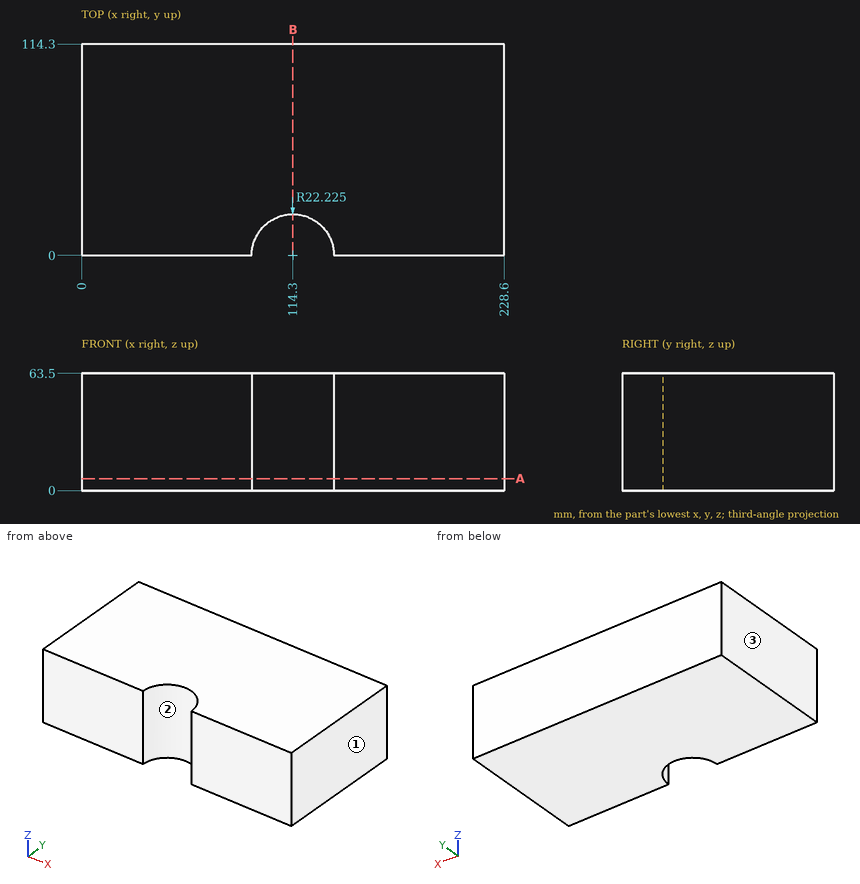
Geometry check sheet. Reference: drawing and pictorial views, mm from the part's lowest x, y, z. Round coordinates to 2 decimals unless told otherwise and drop trailing zeros. Write each loop counter-clockwise with the first axis right and the second up, starting at its lowest first coordinate (ties: lowest second). Pieces come first, ordered by that corner, then holes.
Item 1: Material ranges on line 1 along X through (y, z) = (15, 37); line 2 along X through (y, z) = (5.5, 57); line 3 along Y through (x, z) = (97.5, 31), recorded low to high.
Determined:
line 1: x = 0 to 97.9, 130.7 to 228.6
line 2: x = 0 to 92.77, 135.83 to 228.6
line 3: y = 14.55 to 114.3
Item 2: Go/stop test with a flat-tipped pin: pin 1 Ø1.5 at (x, z) = (108.5, 12.5) entering from -Y. Record where the tip stops, or that it passes through.
Determined:
pin 1: stops at y = 21.24
Item 3: Section check B-B (x = 114.3). Record the boundary of the cut face in (y, z) (3 decimals).
Determined:
outline: (22.225, 0) - (114.3, 0) - (114.3, 63.5) - (22.225, 63.5) - close
Item 4: Section check A-A (z = 6.5). Record the boundary of the cut face in (x, y) (3 decimals), plus the area to 3 significant figures.
Determined:
outline: (0, 0) - (92.075, 0) arc R22.225 cw to (136.525, 0) - (228.6, 0) - (228.6, 114.3) - (0, 114.3) - close
area: 25,400 mm2
Item 5: Mould release check, pull along X, two halves, no side actions. Record for the marked faces 1, 2 and 3: +X half, -X half, draft (parallel to the pull), parting line (faces both ways), or undercut.
Determined:
face 1: +X half
face 2: undercut
face 3: -X half
